Here's how the part is built. I have some questions about the finished solid (model axes, mm). A direction names the side the tool comes from. Coordinates: 2 decimals unless noted, no trailing zeros. Write each loop counter-clockwise with the first axis right and the second up, starting at its lowest first coordinate (ties: lowest second). Pieces come first, ordered by that corner, then holes.
Item 1: Please list where these lines run through material, in increasing order: line 1 (X direction, y = -69, z = 2.8); line 2 (Y direction, x = 0, z = 0.7) (3 decimals); line 3 (Y direction, x = 4.5, z = 2.8).
Item 2: For faces 1 (the face through (-0.16, -57.75, 1.97)), 2 (the face through (-25, -9, 2)), which set-ups out of +Z, -Z, +X, -X, +Y, -Y let a thin tool reach every point of the face, with its end or its side?
Item 3: If we mould it in two halves opening along X, with no side actions, what happens to faces 3 (the face through (-7.25, -78, 2)), 4 (the face through (-20, -110, 2)), 5 (the face through (0, -115, 2))? For each: pulls with the +X half, pulls with the -X half, needs draft (parallel to the pull), parting line crosses it, or undercut.
Item 4: I want a section at A-A (z = 1.7). Please give me the cut outline in (x, y) (3 decimals).
Item 5: I want a section at B-B (x = 0). Please give me the cut outline in (y, z) (3 decimals), and give its area (3 significant figures).
Item 6: I want a section at C-C (x = -20). Please give me the cut outline in (y, z), and give its area (3 significant figures).
from build123d import *

# Parameters (mm, degrees)
BOSS_EXTRUDE1_DEPTH = 4


with BuildPart() as part:
    # Sketch1 → Boss-Extrude1 (new body)
    with BuildSketch(Plane.XY):
        with BuildLine():
            Line((-25, -65), (-25, 90))
            Line((-25, 90), (-9.525, 90))
            ThreePointArc((-9.525, 90), (0, 80.475), (9.525, 90))
            Line((9.525, 90), (25, 90))
            Line((25, 90), (25, -65))
            Line((25, -65), (25, -105))
            Line((25, -105), (15, -115))
            Line((15, -115), (-15, -115))
            Line((-15, -115), (-25, -105))
            Line((-25, -105), (-25, -65))
        make_face()
        with BuildLine():
            Line((-7.25, -90), (-7.25, -65))
            ThreePointArc((-7.25, -65), (0, -57.75), (7.25, -65))
            Line((7.25, -65), (7.25, -90))
            ThreePointArc((7.25, -90), (0, -97.25), (-7.25, -90))
        make_face(mode=Mode.SUBTRACT)
    extrude(amount=BOSS_EXTRUDE1_DEPTH)


solid = part.part
Answer:
1. line 1: x = -25 to -7.25, 7.25 to 25
1. line 2: y = -115 to -97.25, -57.75 to 80.475
1. line 3: y = -115 to -95.68, -59.32 to 81.61
2. face 1: +Z, -Z
2. face 2: +Z, -Z, -X, +Y, -Y
3. face 3: undercut
3. face 4: pulls with the -X half
3. face 5: needs draft
4. outline: (-25, -105) - (-15, -115) - (15, -115) - (25, -105) - (25, 90) - (9.525, 90) arc R9.525 cw to (-9.525, 90) - (-25, 90) - close; hole (-7.25, -90) arc R7.25 ccw to (7.25, -90) - (7.25, -65) arc R7.25 ccw to (-7.25, -65) - close
5. outline: (-115, 0) - (-97.25, 0) - (-97.25, 4) - (-115, 4) - close; (-57.75, 0) - (80.475, 0) - (80.475, 4) - (-57.75, 4) - close
5. area: 624 mm2
6. outline: (-110, 0) - (90, 0) - (90, 4) - (-110, 4) - close
6. area: 800 mm2
